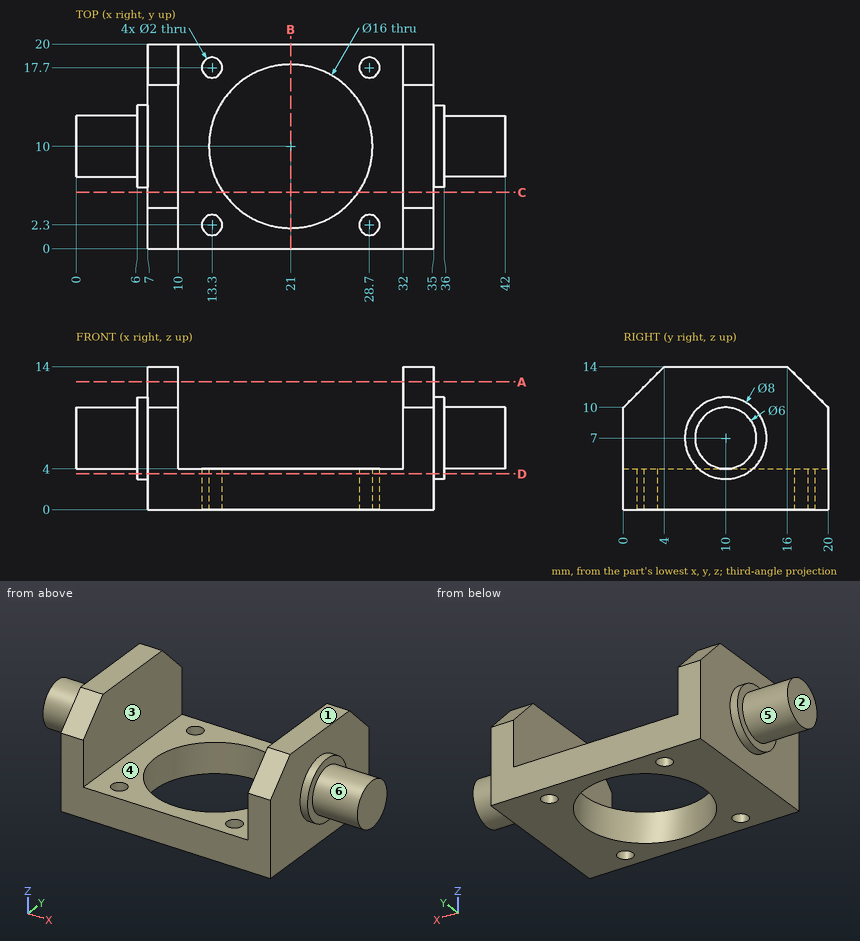
Here's the drawing with two shaded views (mm, measured from the low corner). I have some questions. A direction names the side the tool comes from. Round coordinates to 2 decimals unless told otherwise and drop trailing zeros. Loops run counter-clockwise (first coordinate to the right, second up) from the corner with the lowest first, then second, coordinate; pieces in that order, holes last.
1. For the marked faces 4, 5 and 6, which set-ups out of +Z, -Z, +X, -X, +Y, -Y let a thin tool reach every point of the face, with its end or its side?
Answers:
face 4: +Z, +Y, -Y
face 5: -X
face 6: +X
2. Suppose I cut it at D-D, the plane z = 3.5. Please give me the cut outline in (x, y).
Answers:
outline: (6, 8.06) - (7, 8.06) - (7, 0) - (35, 0) - (35, 8.06) - (36, 8.06) - (36, 11.94) - (35, 11.94) - (35, 20) - (7, 20) - (7, 11.94) - (6, 11.94) - close; hole circle Ø2 at (13.3, 2.3); hole circle Ø2 at (13.3, 17.7); hole circle Ø16 at (21, 10); hole circle Ø2 at (28.7, 2.3); hole circle Ø2 at (28.7, 17.7)
3. Suppose I cut it at B-B, the plane x = 21. Please give me the cut outline in (y, z).
Answers:
outline: (0, 0) - (2, 0) - (2, 4) - (0, 4) - close; (18, 0) - (20, 0) - (20, 4) - (18, 4) - close
4. Suppose I cut it at A-A, the plane z = 12.5. Please give me the cut outline in (x, y), and give its area (3 significant figures).
Answers:
outline: (7, 2.5) - (10, 2.5) - (10, 17.5) - (7, 17.5) - close; (32, 2.5) - (35, 2.5) - (35, 17.5) - (32, 17.5) - close
area: 90.0 mm2
5. Suppose I cut it at C-C, the plane y = 5.5. Please give me the cut outline in (x, z).
Answers:
outline: (7, 0) - (14.39, 0) - (14.39, 4) - (10, 4) - (10, 14) - (7, 14) - close; (27.61, 0) - (35, 0) - (35, 14) - (32, 14) - (32, 4) - (27.61, 4) - close
6. Will these pins go through, and if not, where does the flat tip stop? pin 1 (2 mm diameter, centred on y = 17, z = 5.5, fed in from -X); pin 2 (1 mm diameter, centred on y = 15, z = 6, fed in from +X); pin 3 (4 mm diameter, centred on x = 4.5, z = 9.5, fed in from +Y).
Answers:
pin 1: stops at x = 7
pin 2: stops at x = 35
pin 3: stops at y = 13.82
7. If I drill on probe 1 along X at (y, z) = (10.25, 12.75); probe 2 along X at (y, z) = (9, 6.25); probe 3 along Z at (x, y) = (5, 10), over which ranges is the centre line in solid material (lowest first)?
Answers:
probe 1: x = 7 to 10, 32 to 35
probe 2: x = 0 to 10, 32 to 42
probe 3: z = 4 to 10
8. Thinking about a two-plate mould opening in X: for the marked faces 1, 2 and 3, which applies, released by +X, released by -X, zero draft, split by the parting line, or undercut?
Answers:
face 1: zero draft
face 2: released by -X
face 3: undercut
